The model under review builds one solid part; all positions refer to its coordinate system, in mm. A direction names the side the tool comes from. Coordinates: 2 decimals unless noted, no trailing zeros. Write each loop counter-clockwise with the first axis right and the second up, starting at its lowest first coordinate (ties: lowest second). Pieces come first, ordered by that corner, then holes. Notation, with made-up numbers: (-1, 33) - (51, 33) arc R25 cw to (51, 66) - close; hole circle Ø1 at (-34.75, 74.5). An arc over 180 degrees is marked (long way). Return JSON: item names as keys, results as strings. Group by question number.
(1) We need section B-B on y = 0. State the section outline as (x, z) points, then the cut area to 3 significant figures.
(2) We need section A-A on x = 0. State the section outline as (y, z) points, then the cut area to 3 significant figures.
(3) For pin 1 Ø2 at (x, z) = (-1.5, 5) entering from -Y; pin 2 Ø6 at (y, z) = (0.5, 30.5) entering from -X; pin 3 Ø4 at (x, z) = (-14.5, 2) entering from -Y, all flat-tipped, find the tip position at first contact; note any pin that passes through.
(4) We need section D-D on y = -6. State the section outline as (x, z) points.
(5) Tool access review of faces 1 (the face through (17.264, 5.437, 37.417)), 2 (the face through (0, -7, -19)), 3 (the face through (2.997, -6.61, -11.902)): name each direction out of +Z, -Z, +X, -X, +Y, -Y from which nothing blocks a thin tool from reaching the whole face with its end or side.
(6) We need section C-C on z = 11. State the section outline as (x, y) points, then the cut area to 3 significant figures.
(7) To check wall thickness, follow L1, parallel to Z at x = -8, y = -14.5; L2, parallel to Z at x = 5.5, y = -8.5; L3, parallel to X at y = 0.5, z = 14. State the ranges of each line that lie inside material, in increasing order. Write a range as from..to.
```python
from build123d import *

# Parameters (mm, degrees)
SKETCH1_R           = 18.5
INNER_DEPTH         = 21
SKETCH2_R           = 18.1
OUTER_DEPTH         = 33.3
SKETCH3_R           = 6
BOSS_EXTRUDE3_DEPTH = 5
SKETCH7_R           = 3
BOSS_EXTRUDE6_DEPTH = 14


with BuildPart() as part:
    # Sketch1 → Inner (new body)
    with BuildSketch(Plane.XY):
        with Locations(Location((0, 0, 0), (0, 0, 180))):
            Circle(SKETCH1_R)
    extrude(amount=INNER_DEPTH)

    # Sketch2 → Outer (add)
    with BuildSketch(Plane.XY.offset(21)):
        Circle(SKETCH2_R)
    extrude(amount=OUTER_DEPTH)

    # Sketch3 → Boss-Extrude3 (add)
    with BuildSketch(Plane(origin=(0, 0, 0), x_dir=(-1, 0, 0), z_dir=(0, 0, -1))):
        with Locations(Location((0, -6.742, 0), (0, 0, 180))):
            Circle(SKETCH3_R)
    extrude(amount=BOSS_EXTRUDE3_DEPTH)

    # Sketch7 → Boss-Extrude6 (add)
    with BuildSketch(Plane(origin=(0, 0, -5), x_dir=(-1, 0, 0), z_dir=(0, 0, -1))):
        with Locations((0, -6.742)):
            Circle(SKETCH7_R)
    extrude(amount=BOSS_EXTRUDE6_DEPTH)


solid = part.part
```
Ans:
{
 "1": {"outline": "(-18.5, 0) - (18.5, 0) - (18.5, 21) - (18.1, 21) - (18.1, 54.3) - (-18.1, 54.3) - (-18.1, 21) - (-18.5, 21) - close", "area": "1,980 mm²"},
 "2": {"outline": "(-18.5, 0) - (-12.74, 0) - (-12.74, -5) - (-9.74, -5) - (-9.74, -19) - (-3.74, -19) - (-3.74, -5) - (-0.74, -5) - (-0.74, 0) - (18.5, 0) - (18.5, 21) - (18.1, 21) - (18.1, 54.3) - (-18.1, 54.3) - (-18.1, 21) - (-18.5, 21) - close", "area": "2,130 mm²"},
 "3": {"pin 1": "y = -18.49", "pin 2": "x = -18.1", "pin 3": "y = -13.64"},
 "4": {"outline": "(-17.5, 0) - (-5.95, 0) - (-5.95, -5) - (-2.91, -5) - (-2.91, -19) - (2.91, -19) - (2.91, -5) - (5.95, -5) - (5.95, 0) - (17.5, 0) - (17.5, 21) - (17.08, 21) - (17.08, 54.3) - (-17.08, 54.3) - (-17.08, 21) - (-17.5, 21) - close"},
 "5": {"face 1": "+Z", "face 2": "-Z, +X, -X, +Y, -Y", "face 3": "-Z"},
 "6": {"outline": "circle Ø37 at (0, 0)", "area": "1,080 mm²"},
 "7": {"L1": "0..54.3", "L2": "-5..54.3", "L3": "-18.49..18.49"}
}
